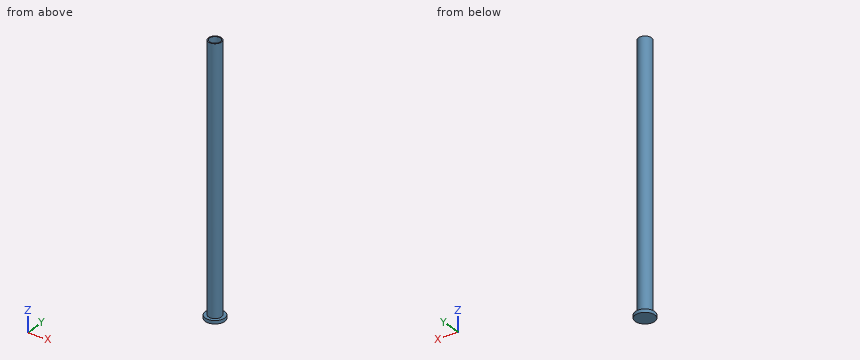
```python
from build123d import *

# Parameters (mm, degrees)
BOSS_EXTRUDE1_DEPTH      = 400
BOSS_EXTRUDE1_DEPTH_BACK = 400
SKETCH3_R                = 20
SKETCH3_R_2              = 17
SKETCH7_R                = 30
BOSS_EXTRUDE4_DEPTH      = 10


with BuildPart() as part:
    # Sketch3 → Boss-Extrude1 (new, two sides: drawn at the far end of the back side and taken through both)
    with BuildSketch(Plane.XY.offset(-BOSS_EXTRUDE1_DEPTH_BACK)):
        Circle(SKETCH3_R)
        Circle(SKETCH3_R_2, mode=Mode.SUBTRACT)
    extrude(amount=BOSS_EXTRUDE1_DEPTH + BOSS_EXTRUDE1_DEPTH_BACK)

    # Sketch7 → Boss-Extrude4 (add)
    with BuildSketch(Plane(origin=(0, 0, -400), x_dir=(-1, 0, 0), z_dir=(0, 0, -1))):
        Circle(SKETCH7_R)
    extrude(amount=BOSS_EXTRUDE4_DEPTH)


solid = part.part
```
Geometry: final body of the model. Coordinates: model frame, mm. Coordinates: 2 decimals unless noted, no trailing zeros. Order: outer loops, then holes, each group sorted by start corner. A loop starts at its lowest first (then second) coordinate and runs counter-clockwise, first axis right, second up. Notation, with made-up numbers: (9.5, -6.75) -> (28.5, -6.75) arc R34 cw to (28.5, 28.25) -> close; hole circle Ø9 at (69, 34). An arc over 180 degrees is marked (long way). Write item = value, one per line.
(1) Line query: line 1 (Y direction, x = 0, z = 80); line 2 (Z direction, x = -13, y = 2); line 3 (Y direction, x = 2, z = 314). Output: solid intervals per line, ascending.
Solved:
line_1 = -20 to -17, 17 to 20
line_2 = -410 to -400
line_3 = -19.9 to -16.88, 16.88 to 19.9
(2) Pin query (flat end, axial travel): pin 1 Ø10 at (x, y) = (-3.5, 7) entering from +Z; pin 2 Ø6 at (x, z) = (-3.5, -35.5) entering from +Y; pin 3 Ø2 at (x, z) = (7.5, -327) entering from +Y; pin 4 Ø2 at (y, z) = (-22, 19.5) entering from +X. Return the tip coordinate at first contact, or that it passes through.
Solved:
pin_1 = -400
pin_2 = 19.99
pin_3 = 18.91
pin_4 = through
(3) Cut plane A-A on y = 0. Return loops of the section in (x, z), plus the area to 3 significant figures.
Solved:
outline = (-30, -410) -> (30, -410) -> (30, -400) -> (20, -400) -> (20, 400) -> (17, 400) -> (17, -400) -> (-17, -400) -> (-17, 400) -> (-20, 400) -> (-20, -400) -> (-30, -400) -> close
area = 5,400 mm²
(4) Cut plane C-C on z = -218. Return loops of the section in (x, y), plus the area to 3 significant figures.
Solved:
outline = circle Ø40 at (0, 0); hole circle Ø34 at (0, 0)
area = 349 mm²
